Build history of the part. All positions in model axes, mm. A direction names the side the tool comes from. Round coordinates to 2 decimals unless told otherwise and drop trailing zeros. Loops run counter-clockwise (first coordinate to the right, second up) from the corner with the lowest first, then second, coordinate; pieces in that order, holes last. Notation, with made-up numbers: (23, 41.5) -> (61, 41.5) arc R25 cw to (61, 68.5) -> close; hole circle Ø9 at (26, 57.25). An arc over 180 degrees is marked (long way). Put each result on its own line as item: value. Start each with the question number.
Item 1: Flat gauge pins, fed straight in: pin 1 Ø3 at (x, z) = (16, 5.5) entering from +Y; pin 2 Ø1 at (y, z) = (-1, -1) entering from +X; pin 3 Ø1.5 at (y, z) = (-0.5, 19.5) entering from +X. Where does each tip first touch, or does it go through?
Item 2: Cut at B-B, the plane y = -6.75. Count the separate pieces of the cut face and the enclosed holes in it, plus the area to 3 significant figures.
Item 3: Cut at C-C, the plane x = -16.2. List the corners of the cut face in (y, z).
Item 4: Pull direction Z, two halves, no side cores. Call faces 3 (the flat face through (-1.4, 10.44, 23.81)), 4 (the flat face through (-8, -9, 16)), 5 (the cylindrical face through (3.5, 10, -1.9)), 6 (the cylindrical face through (17.63, -6.46, 2.59)): +Z half, -Z half, draft (parallel to the pull), parting line (faces both ways), or undercut.
Item 5: Drill centre lines: probe 1 along Y at (x, z) = (-14, 17); probe 2 along X at (y, z) = (-6.75, 22.25); probe 3 along Z at (x, y) = (16.2, -5.95). Where is each one in solid material? Low to high. Write a range as [from, to].
Item 6: Cut at A-A, the plane z = 20.85. List the corners of the cut face in (x, y), plus the area to 3 significant figures.
Item 7: Tool access for faces 1 (the flat face through (-11, -1, 25)), 2 (the flat face through (-12.7, -1, 16)): list every direction of +Z, -Z, +X, -X, +Y, -Y with a clear straight run to the whole face (end or side of a thin tool).
```python
from build123d import *

# Parameters (mm, degrees)
F0_W          = 7
F0_H          = 5
F1_DEPTH      = 25
F1_DEPTH_BACK = 2
F4_DEPTH      = 25
F4_DEPTH_BACK = 25
F5_DEPTH      = 25
F5_DEPTH_BACK = 25
F6_R          = 1
F7_R          = 1.75
F7_R_2        = 1.5
F8_DEPTH      = 25
F9_T1_DEPTH   = 20
F9_T3_DEPTH   = 13.6602540378
F9_T5_DEPTH   = 8.256448117
F9_T7_DEPTH   = 5.0368572892


# Not quite as in the source:
# - a fillet or chamfer that OpenCascade refuses, or shapes differently, is made with other operations: its cross-section is extruded or revolved along the edge and cut away or added


with BuildPart() as f1:
    # F0 (on Top) → F1 (new body, two sides)
    with BuildSketch(Plane.XY) as f1_sk:
        with Locations((-16.2, -6.5)):
            Rectangle(F0_W, F0_H)
        with Locations((16.2, -6.5)):
            Rectangle(F0_W, F0_H)
        with BuildLine():
            ThreePointArc((-12.0536301586, -4), (-12.5373662109, -2.0259438524), (-12.7, 0))
            Line((-12.7, 0), (-12.7, -4))
            Line((-12.7, -4), (-12.0536301586, -4))
        make_face()
        with BuildLine():
            Line((12.7, -4), (12.7, 0))
            ThreePointArc((12.7, 0), (12.5373662109, -2.0259438524), (12.0536301586, -4))
            Line((12.0536301586, -4), (12.7, -4))
        make_face()
        with BuildLine():
            ThreePointArc((-8.7, 0), (0, 8.7), (8.7, 0))
            Line((8.7, 0), (12.7, 0))
            ThreePointArc((12.7, 0), (0, 12.7), (-12.7, 0))
            Line((-12.7, 0), (-8.7, 0))
        make_face()
        with BuildLine():
            ThreePointArc((-8.9604687377, -9), (-10.8003744429, -6.6814603115), (-12.0536301586, -4))
            Line((-12.0536301586, -4), (-12.7, -4))
            Line((-12.7, -4), (-12.7, -9))
            Line((-12.7, -9), (-8.9604687377, -9))
        make_face()
        with BuildLine():
            Line((12.7, -4), (12.0536301586, -4))
            ThreePointArc((12.0536301586, -4), (10.8003744429, -6.6814603115), (8.9604687377, -9))
            Line((8.9604687377, -9), (12.7, -9))
            Line((12.7, -9), (12.7, -4))
        make_face()
        with BuildLine():
            ThreePointArc((-7.7259303647, -4), (-8.452975635, -2.0584467235), (-8.7, 0))
            Line((-8.7, 0), (-12.7, 0))
            ThreePointArc((-12.7, 0), (-12.5373662109, -2.0259438524), (-12.0536301586, -4))
            Line((-12.0536301586, -4), (-7.7259303647, -4))
        make_face()
        with BuildLine():
            Line((12.7, 0), (8.7, 0))
            ThreePointArc((8.7, 0), (8.452975635, -2.0584467235), (7.7259303647, -4))
            Line((7.7259303647, -4), (12.0536301586, -4))
            ThreePointArc((12.0536301586, -4), (12.5373662109, -2.0259438524), (12.7, 0))
        make_face()
        with BuildLine():
            ThreePointArc((-1, -8.6423376467), (-4.9419925019, -7.1600775213), (-7.7259303647, -4))
            Line((-7.7259303647, -4), (-12.0536301586, -4))
            ThreePointArc((-12.0536301586, -4), (-10.8003744429, -6.6814603115), (-8.9604687377, -9))
            Line((-8.9604687377, -9), (-1, -9))
            Line((-1, -9), (-1, -8.6423376467))
        make_face()
        with BuildLine():
            Line((12.0536301586, -4), (7.7259303647, -4))
            ThreePointArc((7.7259303647, -4), (4.9419925019, -7.1600775213), (1, -8.6423376467))
            Line((1, -8.6423376467), (1, -9))
            Line((1, -9), (8.9604687377, -9))
            ThreePointArc((8.9604687377, -9), (10.8003744429, -6.6814603115), (12.0536301586, -4))
        make_face()
    extrude(amount=F1_DEPTH)
    extrude(f1_sk.sketch, amount=-F1_DEPTH_BACK)

    # F3 (on Front) → F4 (cut, two sides)
    with BuildSketch(Plane.XZ) as f4_sk:
        Polygon((0.0041016151, 23), (0, 23), (39.8371685741, 0), (39.8371685741, 23), (28.9984290028, 23), (28.9984290028, 6.2601172778), align=None)
        Polygon((-3.46, 25), (0.0041016151, 23), (28.9984290028, 23), (28.9984290028, 25), align=None)
        Polygon((28.9984290028, 23), (0.0041016151, 23), (28.9984290028, 6.2601172778), align=None)
    extrude(amount=F4_DEPTH, mode=Mode.SUBTRACT)
    extrude(f4_sk.sketch, amount=-F4_DEPTH_BACK, mode=Mode.SUBTRACT)

    # F2 (on Front) → F5 (cut, two sides)
    with BuildSketch(Plane.XZ) as f5_sk:
        Polygon((-0.0041016151, 0), (0, 0), (-8.2087842873, 4.739343818), (-8.2087842873, 4.7369757494), align=None)
        Polygon((3.46, -2), (-0.0041016151, 0), (-8.2087842873, 0), (-8.2087842873, 4.7369757494), (-21.54, 12.4337567297), (-21.54, -2), align=None)
        Polygon((-8.2087842873, 0), (-0.0041016151, 0), (-8.2087842873, 4.7369757494), align=None)
    extrude(amount=F5_DEPTH, mode=Mode.SUBTRACT)
    extrude(f5_sk.sketch, amount=-F5_DEPTH_BACK, mode=Mode.SUBTRACT)

    # F6
    f6_edges = [f1.edges().sort_by_distance(p)[0] for p in [
        (12.7, -4, 6.833826),
        (-12.7, -4, 16.16499),
    ]]
    fillet(f6_edges, radius=F6_R)

    # F7 (on Front) → F8 (cut)
    with BuildSketch(Plane.XZ):
        with Locations((-16.2, 20.85)):
            Circle(F7_R)
        with Locations((16.2, 2.14)):
            Circle(F7_R_2)
    extrude(amount=F8_DEPTH, mode=Mode.SUBTRACT)

    # F9: fillet of radius 3 on 8 edges, made by hand

    # F9_s2 → F9_t1 (cut)
    with BuildSketch(Plane.XZ.offset(-3.5)):
        with BuildLine():
            ThreePointArc((16.7, -2), (18.8213203436, -1.1213203436), (19.7, 1))
            Line((19.7, 1), (19.7, -2))
            Line((19.7, -2), (16.7, -2))
        make_face()
        with BuildLine():
            ThreePointArc((-19.7, 22), (-18.8213203436, 24.1213203436), (-16.7, 25))
            Line((-16.7, 25), (-19.7, 25))
            Line((-19.7, 25), (-19.7, 22))
        make_face()
    extrude(amount=F9_T1_DEPTH, mode=Mode.SUBTRACT)

    # F9_s4 → F9_t3 (cut)
    with BuildSketch(Plane.XZ.offset(-0.3301270189)):
        with BuildLine():
            ThreePointArc((18.2, 12.4922251007), (19.2980762114, 11.3941488894), (19.7, 9.8941488894))
            Line((19.7, 9.8941488894), (19.7, 11.626199697))
            Line((19.7, 11.626199697), (18.2, 12.4922251007))
        make_face()
        with BuildLine():
            ThreePointArc((-18.2, 10.5054068306), (-19.2980762114, 11.603483042), (-19.7, 13.103483042))
            Line((-19.7, 13.103483042), (-19.7, 11.3714322344))
            Line((-19.7, 11.3714322344), (-18.2, 10.5054068306))
        make_face()
    extrude(amount=F9_T3_DEPTH, mode=Mode.SUBTRACT)

    # F9_s6 → F9_t5 (cut)
    with BuildSketch(Plane.XZ.offset(-14.2292097711)):
        with BuildLine():
            ThreePointArc((-4.2638475773, 25), (-3.487390442, 24.8977774789), (-2.7638475773, 24.5980762114))
            Line((-2.7638475773, 24.5980762114), (-3.46, 25))
            Line((-3.46, 25), (-4.2638475773, 25))
        make_face()
        with BuildLine():
            ThreePointArc((4.2638475773, -2), (3.487390442, -1.8977774789), (2.7638475773, -1.5980762114))
            Line((2.7638475773, -1.5980762114), (3.46, -2))
            Line((3.46, -2), (4.2638475773, -2))
        make_face()
    extrude(amount=F9_T5_DEPTH, mode=Mode.SUBTRACT)

    # F9_s8 → F9_t7 (cut)
    with BuildSketch(Plane.XZ.offset(5.9727616541)):
        with BuildLine():
            ThreePointArc((4.2638475773, -2), (3.487390442, -1.8977774789), (2.7638475773, -1.5980762114))
            Line((2.7638475773, -1.5980762114), (3.46, -2))
            Line((3.46, -2), (4.2638475773, -2))
        make_face()
        with BuildLine():
            ThreePointArc((-4.2638475773, 25), (-3.487390442, 24.8977774789), (-2.7638475773, 24.5980762114))
            Line((-2.7638475773, 24.5980762114), (-3.46, 25))
            Line((-3.46, 25), (-4.2638475773, 25))
        make_face()
    extrude(amount=F9_T7_DEPTH, mode=Mode.SUBTRACT)


solid = f1.part
```
Reply:
1. pin 1: stops at y = -4
1. pin 2: stops at x = 12.7
1. pin 3: stops at x = -8.61
2. separate pieces: 2
2. enclosed holes: 2
2. area: 482 mm^2
3. outline: (-9, 9.35) -> (-4, 9.35) -> (-4, 19.1) -> (-9, 19.1) -> close; (-9, 22.6) -> (-4, 22.6) -> (-4, 25) -> (-9, 25) -> close
4. face 3: +Z half
4. face 4: draft
4. face 5: -Z half
4. face 6: undercut
5. probe 1: y = [-9, -4]
5. probe 2: x = [-19.69, -17.25], [-15.15, -5.49]
5. probe 3: z = [-2, 0.64], [3.64, 13.65]
6. outline: (-19.7, -9) -> (-17.95, -9) -> (-17.95, -4) -> (-19.7, -4) -> close; (-14.45, -9) -> (-1, -9) -> (-1, -8.64) arc R8.7 cw (long way) to (3.72, 7.86) -> (3.72, 12.14) arc R12.7 ccw to (-12.7, 0) -> (-12.7, -3) arc R1 cw to (-13.7, -4) -> (-14.45, -4) -> close; (1, -9) -> (3.72, -9) -> (3.72, -7.86) arc R8.7 cw to (1, -8.64) -> close
6. area: 157 mm^2
7. face 1: +Z, +X, -X, +Y, -Y
7. face 2: +Z, -Z, -X, +Y
